Geometry: final body of the model. Coordinates: model frame, mm. Face numbers are marked on the shaded views. A direction names the side the tool comes from. Give positions to 0.01 mm unless a question says otherwise; leave off trailing zeros. Write each loop counter-clockwise with the first axis right and the second up, starting at its lowest first coordinate (ties: lowest second). Pieces come first, ordered by that corner, then holes.
Q1. Reachability of the marked faces 4, 5 and 6 from +Z, -Z, +X, -X, +Y, -Y: full face, straight path, thin tool, end or side. Return the list, or none.
Q2. Pin query (flat end, axial travel): pin 1 (23 mm diameter, centred on y = 80, z = 0, fed in from +X); pin 2 (3 mm diameter, centred on x = 19.5, y = -6.5, fed in from +Z); pin 3 (1.5 mm diameter, centred on x = 37, z = -23, fed in from -Y); pin 4 (12 mm diameter, centred on x = 8.5, z = -16, fed in from -Y). Return the tip coordinate at first contact, or that it passes through.
Q3. Draft query along Z for the marked faces 1, 2 and 3. Return one class per face: pulls with the +Z half, pulls with the -Z half, needs draft (parallel to the pull), parting line crosses it, or undercut.
Q4. Cut plane C-C on x = 34. Return the cut outline in (y, z).
Q5. Cut plane A-A on x = 44.5. Return the cut outline in (y, z).
Q6. Line query: L1, parallel to Y at x = 16, z = -1; L2, parallel to Y at x = 16, z = 2; L3, parallel to X at y = 91.5, z = 10.5. Output: solid intervals per line, ascending.
Q7. Cut plane D-D on y = 0. Return the cut outline in (x, z), plus the area to 3 significant figures.
Q8. Cut plane B-B on z = 0. Return the cut outline in (x, y).
Autodesk Inventor part; units mm, degrees
ref_plane "Work Plane1" through (25, 0, 0) normal (1, 0, 0) x (0, 0, -1)
ref_plane "YZ Plane" through (0, 0, 0) normal (1, 0, 0) x (0, 1, 0)
ref_plane "XZ Plane" through (0, 0, 0) normal (0, 1, 0) x (-1, 0, 0)
sketch "Sketch1" plane through (0, 0, 0) normal (1, 0, 0) x (0, 1, 0)
  circle A0 centre (0, 0) radius 30
  circle A1 centre (0, 0) radius 16
  dimension "d0" = 60
  dimension "d1" = 32
extrude "Extrusion1" add sketch "Sketch1" along normal blind 50
sketch "Sketch2" plane through (50, 0, 0) normal (1, 0, 0) x (0, 0, -1)
  circle A0 centre (0, 80) radius 10
  circle A1 centre (0, 80) radius 20
  line L0 (-19.8431, 82.5) -> (-29.7647, 3.75)
  line L1 (19.8431, 82.5) -> (29.7647, 3.75)
  circle A2 centre (0, 0) radius 30
  line L2 (-25.1976, 40) -> (25.1976, 40)
  dimension "d4" = 20
  dimension "d5" = 40
  dimension "d6" = 80
  dimension "d7" = 40
extrude "Extrusion2" add sketch "Sketch2" against normal blind 50 contours A1 | A1 L1 L2 L0
sketch "Sketch3" plane through (0, 0, 0) normal (0, 0, 1) x (1, 0, 0)
  line L0 (12.5, 115.7738) -> (37.5, 115.7738)
  line L1 (37.5, 115.7738) -> (37.5, 55.7738)
  line L2 (37.5, 55.7738) -> (12.5, 55.7738)
  line L3 (12.5, 55.7738) -> (12.5, 115.7738)
  line L4 (0, 100) -> (0, 82.5)
  line L5 (0, 70) -> (0, 90)
  line L6 (50, 90) -> (50, 70)
  line L7 (0, 80.7738) -> (50, 80.7738)
  point P0 (0, 0)
  dimension "d10" = 12.5
  dimension "d11" = 25
  dimension "d12" = 25
  dimension "d13" = 60
extrude "Extrusion3" cut sketch "Sketch3" along normal through all both and the other way through all
ref_plane "Work Plane1" through (25, 0, 0) normal (1, 0, 0) x (0, 0, -1)
sketch "Sketch4" plane through (25, 0, 0) normal (1, 0, 0) x (0, 0, -1)
  line L0 (25.1976, 40) -> (29.7647, 3.75)
  line L1 (-25.1976, 40) -> (-29.7647, 3.75)
  circle A0 centre (0, 0) radius 30
  line L2 (25.1976, 40) -> (-25.1976, 40)
extrude "Extrusion4" add sketch "Sketch4" along normal mid plane 15 contours L0 A0 L1 L2
properties part number "Exercise04"
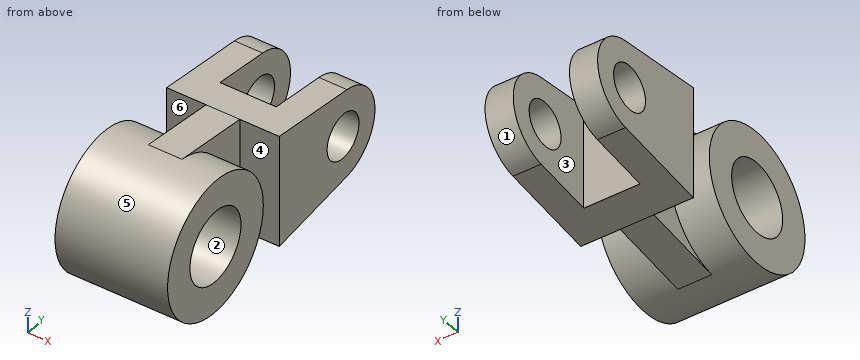
Data:
1. face 4: +Z, -Z, +X
1. face 5: none
1. face 6: +Z, -Z, -X
2. pin 1: stops at x = 50
2. pin 2: stops at z = 29.58
2. pin 3: stops at y = -20.12
2. pin 4: stops at y = -28.28
3. face 1: parting line crosses it
3. face 2: undercut
3. face 3: needs draft
4. outline: circle Ø60 at (0, 0); (40, -25.2) - (55.77, -23.21) - (55.77, 23.21) - (40, 25.2) - close; hole circle Ø32 at (0, 0)
5. outline: circle Ø60 at (0, 0); (40, -25.2) - (82.5, -19.84) arc R20 ccw to (82.5, 19.84) - (40, 25.2) - close; hole circle Ø32 at (0, 0); hole circle Ø20 at (80, 0)
6. L1: y = -29.98 to -15.97, 15.97 to 29.98, 40 to 55.77
6. L2: y = -29.93 to -15.87, 15.87 to 29.93, 40 to 55.77
6. L3: x = 0 to 12.5, 37.5 to 50
7. outline: (0, -30) - (50, -30) - (50, -16) - (0, -16) - close; (0, 16) - (50, 16) - (50, 30) - (0, 30) - close
7. area: 1,400 mm2
8. outline: (0, -30) - (50, -30) - (50, -16) - (0, -16) - close; (0, 16) - (50, 16) - (50, 30) - (32.5, 30) - (32.5, 40) - (50, 40) - (50, 70) - (37.5, 70) - (37.5, 55.77) - (12.5, 55.77) - (12.5, 70) - (0, 70) - (0, 40) - (17.5, 40) - (17.5, 30) - (0, 30) - close; (0, 90) - (12.5, 90) - (12.5, 100) - (0, 100) - close; (37.5, 90) - (50, 90) - (50, 100) - (37.5, 100) - close
